Input: part model. Units: mm. Frame: model coordinates. A direction names the side the tool comes from. Coordinates: 2 decimals unless noted, no trailing zeros. Write each loop counter-clockwise with the first axis right and the second up, starting at its lowest first coordinate (ties: lowest second). Pieces come first, ordered by that corner, then holes.
1) Draft query along Y for faces 1 (the cylindrical face through (25, 9.8, -41.1)), 2 (the cylindrical face through (25.756, 15.278, 43.689)), 3 (the flat face through (25, 3.002, -39)), 4 (the flat face through (25, -1, -44.452)). Return one class per face: pulls with the +Y half, pulls with the -Y half, needs draft (parallel to the pull), parting line crosses it, or undercut.
2) Set-up query: faces 5 (the cylindrical face through (25.756, 3.726, -34.216)), 6 (the flat face through (25, -1, 44.452)). Return all of +Z, -Z, +X, -X, +Y, -Y with unobstructed straight access to the full face (end or side cutting, diameter ignored); none if empty.
3) Section query C-C (z = -25). Output: boundary loops of the cut face in (x, y).
4) Section query A-A (y = -1). Output: boundary loops of the cut face in (x, z).
5) Section query D-D (y = 4). Output: boundary loops of the cut face in (x, z).
6) Line query: L1, parallel to Z at x = 31, y = 6.5; L2, parallel to Z at x = 14.5, y = 0; L3, parallel to Y at x = 36.5, z = -38. Output: solid intervals per line, ascending.
7) Pin query (flat end, axial travel): pin 1 Ø10 at (y, z) = (11.5, -22.5) entering from -X; pin 2 Ø5.5 at (y, z) = (9.65, 38.1) entering from +X; pin 3 Ø3 at (x, z) = (25, 38.5) entering from -Y; pin 4 Ø2 at (x, z) = (21, 11.5) entering from -Y. Return the tip coordinate at first contact, or that it passes through.
8) Section query B-B (x = 47). Output: boundary loops of the cut face in (y, z), then the cut area to 3 significant figures.
from build123d import *

# Parameters (mm, degrees)
SKETCH1_W           = 88.905
SKETCH1_H           = 32.004
BOSS_EXTRUDE1_DEPTH = 50.8
FILLET1_R           = 2.54
FILLET2_R           = 2.54
SKETCH13_W          = 83.825
SKETCH13_H          = 29.464
CUT_EXTRUDE1_DEPTH  = 90
SKETCH15_W          = 8.46
SKETCH15_H          = 10.46
SKETCH15_R          = 3
BOSS_EXTRUDE8_DEPTH = 50.8
SKETCH19_W          = 8.46
SKETCH19_H          = 10.46
SKETCH19_R          = 3
BOSS_EXTRUDE9_DEPTH = 50.8
FILLET3_R           = 2.54


with BuildPart() as part:
    # Sketch1 → Boss-Extrude1 (new body)
    with BuildSketch(Plane(origin=(0, 0, 0), x_dir=(0, 0, -1), z_dir=(1, 0, 0))):
        Rectangle(SKETCH1_W, SKETCH1_H)
    extrude(amount=BOSS_EXTRUDE1_DEPTH)

    # Fillet1
    fillet1_edges = [part.edges().sort_by_distance(p)[0] for p in [
        (25.4, 16.002, -44.4525),
    ]]
    fillet(fillet1_edges, radius=FILLET1_R)

    # Fillet2
    fillet2_edges = [part.edges().sort_by_distance(p)[0] for p in [
        (25.4, 16.002, 44.4525),
    ]]
    fillet(fillet2_edges, radius=FILLET2_R)

    # Sketch13 → Cut-Extrude1 (cut)
    with BuildSketch(Plane.ZY):
        with Locations((0, -1.27)):
            Rectangle(SKETCH13_W, SKETCH13_H)
    extrude(amount=-CUT_EXTRUDE1_DEPTH, mode=Mode.SUBTRACT)

    # Sketch15 → Boss-Extrude8 (add)
    with BuildSketch(Plane.ZY):
        with Locations((37.6825, 8.232)):
            Rectangle(SKETCH15_W, SKETCH15_H)
        with Locations((38.1025, 9.652)):
            Circle(SKETCH15_R, mode=Mode.SUBTRACT)
    extrude(amount=-BOSS_EXTRUDE8_DEPTH)

    # Sketch19 → Boss-Extrude9 (add)
    with BuildSketch(Plane.ZY):
        with Locations((-37.6825, 8.232)):
            Rectangle(SKETCH19_W, SKETCH19_H)
        with Locations((-38.1025, 9.652)):
            Circle(SKETCH19_R, mode=Mode.SUBTRACT)
    extrude(amount=-BOSS_EXTRUDE9_DEPTH)

    # Fillet3
    fillet3_edges = [part.edges().sort_by_distance(p)[0] for p in [
        (25.4, 3.002, 33.4525),
        (25.4, 3.002, -33.4525),
    ]]
    fillet(fillet3_edges, radius=FILLET3_R)


solid = part.part
Answer:
1. face 1: undercut
1. face 2: pulls with the +Y half
1. face 3: pulls with the -Y half
1. face 4: needs draft
2. face 5: +X, -X, -Y
2. face 6: +Z, +X, -X, +Y, -Y
3. outline: (0, 13.46) - (50.8, 13.46) - (50.8, 16) - (0, 16) - close
4. outline: (0, -44.45) - (50.8, -44.45) - (50.8, -41.91) - (0, -41.91) - close; (0, 41.91) - (50.8, 41.91) - (50.8, 44.45) - (0, 44.45) - close
5. outline: (0, -44.45) - (50.8, -44.45) - (50.8, -33.97) - (0, -33.97) - close; (0, 33.97) - (50.8, 33.97) - (50.8, 44.45) - (0, 44.45) - close
6. L1: z = -44.45 to -33.45, 33.45 to 44.45
6. L2: z = -44.45 to -41.91, 41.91 to 44.45
6. L3: y = 3 to 6.65, 12.65 to 16
7. pin 1: stops at x = 0
7. pin 2: passes through
7. pin 3: stops at y = 3
7. pin 4: stops at y = 13.46
8. outline: (-16, -44.45) - (13.46, -44.45) arc R2.54 ccw to (16, -41.91) - (16, 41.91) arc R2.54 ccw to (13.46, 44.45) - (-16, 44.45) - (-16, 41.91) - (3, 41.91) - (3, 35.99) arc R2.54 ccw to (5.54, 33.45) - (13.46, 33.45) - (13.46, -33.45) - (5.54, -33.45) arc R2.54 ccw to (3, -35.99) - (3, -41.91) - (-16, -41.91) - close; hole circle Ø6 at (9.65, -38.1); hole circle Ø6 at (9.65, 38.1)
8. area: 490 mm2
